The listing builds one solid part. Answer for the finished solid, in the listing's coordinates (mm). A direction names the side the tool comes from. Coordinates: 2 decimals unless noted, no trailing zeros. Write each loop counter-clockwise with the first axis right and the second up, starting at its lowest first coordinate (ties: lowest second). Pieces come first, ordered by that corner, then holes. Notation, with made-up numbers: M 6,-11 L 52,-11 A21 cw 52,12 Z; hole C -38,76 d11. An arc over 180 degrees is marked long. Write item = value, one per line. Start each with the question number.
```python
from build123d import *

# Parameters (mm, degrees)
SKETCH1_W           = 75
SKETCH1_H           = 77
BOSS_EXTRUDE1_DEPTH = 3.2
SKETCH2_W           = 3
SKETCH2_H           = 11
BOSS_EXTRUDE3_DEPTH = 3.2
LPATTERN1_COUNT     = 4
LPATTERN1_PITCH     = 22
SKETCH5_W           = 14
SKETCH5_H           = 2.85
SKETCH5_W_2         = 2.3
SKETCH5_H_2         = 6.3
CUT_EXTRUDE1_DEPTH  = 56.970885289
LPATTERN3_COUNT     = 3
LPATTERN3_PITCH     = 22
SKETCH4_W           = 3
SKETCH4_H           = 11
BOSS_EXTRUDE6_DEPTH = 3.2
SKETCH7_R           = 1.44
CUT_EXTRUDE2_DEPTH  = 56.970885289
LPATTERN7_COUNT     = 3
LPATTERN7_PITCH     = 22
LPATTERN8_COUNT     = 3
LPATTERN8_PITCH     = 22


with BuildPart() as part:
    # Sketch1 → Boss-Extrude1 (new body)
    with BuildSketch(Plane(origin=(0, 0, 0), x_dir=(1, 0, 0), z_dir=(0, 1, 0))):
        Rectangle(SKETCH1_W, SKETCH1_H)
    extrude(amount=BOSS_EXTRUDE1_DEPTH)

    # Sketch2 → Boss-Extrude3 (add)
    with BuildSketch(Plane(origin=(0, 3.2, 0), x_dir=(1, 0, 0), z_dir=(0, 1, 0))):
        with Locations((-39, 33)):
            Rectangle(SKETCH2_W, SKETCH2_H)
    boss_extrude3 = extrude(amount=-BOSS_EXTRUDE3_DEPTH)

    # LPattern1: Boss-Extrude3 ×4
    with Locations(*[(0, 0, i * LPATTERN1_PITCH) for i in range(1, LPATTERN1_COUNT)]):
        add(boss_extrude3)

    # Sketch5 → Cut-Extrude1 (cut, through all)
    with BuildSketch(Plane(origin=(0, 3.2, 0), x_dir=(1, 0, 0), z_dir=(0, 1, 0))):
        with Locations((-30.5, 22)):
            Rectangle(SKETCH5_W, SKETCH5_H)
        with Locations((-30.5, 22)):
            Rectangle(SKETCH5_W_2, SKETCH5_H_2)
    cut_extrude1 = extrude(amount=-CUT_EXTRUDE1_DEPTH, mode=Mode.SUBTRACT)

    # LPattern3: Cut-Extrude1 ×3
    with Locations(*[(0, 0, i * LPATTERN3_PITCH) for i in range(1, LPATTERN3_COUNT)]):
        add(cut_extrude1, mode=Mode.SUBTRACT)

    # Sketch4 → Boss-Extrude6 (add)
    with BuildSketch(Plane(origin=(0, 3.2, 0), x_dir=(1, 0, 0), z_dir=(0, 1, 0))):
        with Locations((39, 22)):
            Rectangle(SKETCH4_W, SKETCH4_H)
    boss_extrude6 = extrude(amount=-BOSS_EXTRUDE6_DEPTH)

    # Sketch7 → Cut-Extrude2 (cut, through all)
    with BuildSketch(Plane(origin=(0, 3.2, 0), x_dir=(1, 0, 0), z_dir=(0, 1, 0))):
        with Locations(Location((38.06, 22, 0), (0, 0, 270))):
            Circle(SKETCH7_R)
    cut_extrude2 = extrude(amount=-CUT_EXTRUDE2_DEPTH, mode=Mode.SUBTRACT)

    # LPattern7: Boss-Extrude6 ×3
    with Locations(*[(0, 0, i * LPATTERN7_PITCH) for i in range(1, LPATTERN7_COUNT)]):
        add(boss_extrude6)

    # LPattern8: Cut-Extrude2 ×3
    with Locations(*[(0, 0, i * LPATTERN8_PITCH) for i in range(1, LPATTERN8_COUNT)]):
        add(cut_extrude2, mode=Mode.SUBTRACT)


solid = part.part
```
1. The part is cut by section C-C, the plane y = 0.95. Count the separate pieces of the cut face and the enclosed holes in it, and give its area (3 significant figures).
2. Each of these flat-tipped pins is pushed along its axis until it touches: pin 1 (1.5 mm diameter, centred on y = 1, z = -1.5, fed in from -X); pin 2 (12 mm diameter, centred on x = 8, z = -21, fed in from -Y); pin 3 (2.5 mm diameter, centred on x = 38.06, z = -22, fed in from +Y). Where does it stop, or does it pass through?
3. For faces 4 (the face through (-40.5, 2, -33)), 5 (the face through (39, 2, -5.5)), 6 (the face through (39, 2, 27.5)), 7 (the face through (-29.35, 2, -20)), 8 (the face through (-35, 2, 20.575)), determine the directions among +Z, -Z, +X, -X, +Y, -Y from which every point of the face is accessible in a straight line to the end or side of a thin tool.
4. The part is cut by section D-D, the plane z = -0.5. Write down the section's boundary in (x, y).
5. Straight lines are drawn through the part: L1, parallel to X at y = 1.4, z = 22; L2, parallel to X at y = 2.2, z = 3; L3, parallel to X at y = 1.4, z = -31. For each, find the intervals that lie inside material, in ascending order. Write a range as [from, to].
6. The part is cut by section B-B, the plane x = -33. Write down the section's boundary in (y, z) (3 decimals), and give its area (3 significant figures).
7. The part is cut by section A-A, the plane z = 22. Write down the section's boundary in (x, y), and give its area (3 significant figures).
8. For a pull along X with two mould halves and no side action, classify faces 1 (the face through (-39, 2, 27.5)), 2 (the face through (-31, 2, -25.15)), 3 (the face through (-37.5, 2, -3)) as pulls with the +X half, pulls with the -X half, needs draft (parallel to the pull), parting line crosses it, or undercut.
Solution:
q1.separate_pieces = 1
q1.enclosed_holes = 3
q1.area = 5,840 mm^2
q2.pin_1 = -37.5
q2.pin_2 = 0
q2.pin_3 = through
q3.face_4 = +Z, -Z, -X, +Y, -Y
q3.face_5 = +X, +Y, -Y
q3.face_6 = +Z, +X, +Y, -Y
q3.face_7 = +Y, -Y
q3.face_8 = -X, +Y, -Y
q4.outline = M -23.5,0 L 36.71,0 L 36.71,3.2 L -23.5,3.2 Z; M 39.41,0 L 40.5,0 L 40.5,3.2 L 39.41,3.2 Z
q5.L1 = [-23.5, 36.62], [39.5, 40.5]
q5.L2 = [-37.5, -31.65], [-29.35, 40.5]
q5.L3 = [-40.5, 37.5]
q6.outline = M 0,-38.5 L 3.2,-38.5 L 3.2,-23.425 L 0,-23.425 Z; M 0,-20.575 L 3.2,-20.575 L 3.2,-1.425 L 0,-1.425 Z; M 0,1.425 L 3.2,1.425 L 3.2,20.575 L 0,20.575 Z; M 0,23.425 L 3.2,23.425 L 3.2,38.5 L 0,38.5 Z
q6.area = 219 mm^2
q7.outline = M -23.5,0 L 36.62,0 L 36.62,3.2 L -23.5,3.2 Z; M 39.5,0 L 40.5,0 L 40.5,3.2 L 39.5,3.2 Z
q7.area = 196 mm^2
q8.face_1 = needs draft
q8.face_2 = undercut
q8.face_3 = pulls with the -X half
